Source: CAD feature listing. Evaluate the final solid. Frame: model axes, mm. Give positions to 0.01 mm unless a question says otherwise; leave off trailing zeros. Order: outer loops, then holes, each group sorted by start corner. A loop starts at its lowest first (then second) coordinate and runs counter-clockwise, first axis right, second up. Notation, with made-up numbers: (66, 66.25) -> (103, 66.25) arc R18 ccw to (103, 83.25) -> close; hole circle Ø11 at (29.5, 88.25). An arc over 180 degrees is marked (long way). Answer in a Markdown table with one row per item.
Solid Edge part; units mm, degrees
sketch "Sketch1" plane through (0, 0, 0) normal (0, 0, 1) x (1, 0, 0)
  line L0 (-52, -100) -> (52, -100)
  line L1 (52, -100) -> (52, 100)
  line L2 (52, 100) -> (-52, 100)
  line L3 (-52, 100) -> (-52, -100)
  line L4 (-25, -66) -> (25, -66)
  arc A0 (25, -66) -> (27, -64) centre (25, -64) ccw
  line L5 (27, -64) -> (27, 64)
  arc A1 (27, 64) -> (25, 66) centre (25, 64) ccw
  line L6 (25, 66) -> (-25, 66)
  arc A2 (-25, 66) -> (-27, 64) centre (-25, 64) ccw
  line L7 (-27, 64) -> (-27, -64)
  arc A3 (-25, -66) -> (-27, -64) centre (-25, -64) cw
extrude "Extrusionsausprägung_1" add sketch "Sketch1" along normal blind 2.5
hole "Bohrung_1" at (-44.9, 90, 2.5) direction (0, 0, -1) diameter 7.1 end up to next
hole "Hole1" at (44.9, 90, 2.5) direction (0, 0, -1) diameter 7.1 end up to next
hole "Hole2" at (44.9, -90, 2.5) direction (0, 0, -1) diameter 7.1 end up to next
hole "Hole3" at (-44.9, -90, 2.5) direction (0, 0, -1) diameter 7.1 end up to next
hole "Bohrung_5" at (44.9, 0, 2.5) direction (0, 0, -1) diameter 3.3 end up to next countersink diameter 6.3 countersink angle 120
hole "Hole4" at (-44.9, 0, 2.5) direction (0, 0, -1) diameter 3.3 end up to next countersink diameter 6.3 countersink angle 120
properties material "Aluminium, 2024-T4"
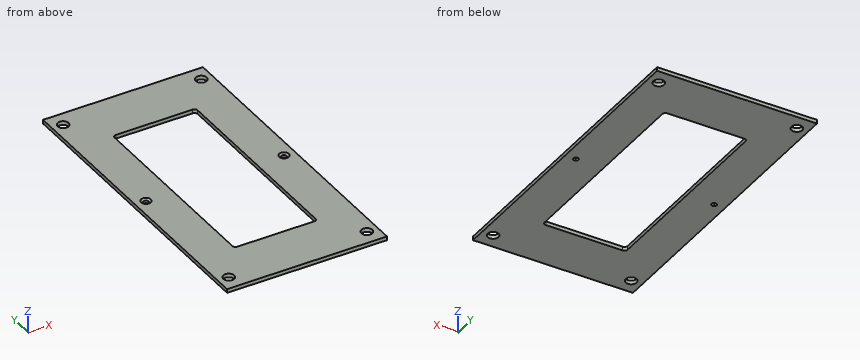
(1) Ray query, probe 1 along Y at (x, z) = (44.9, 1.3); probe 2 along X at (y, z) = (-90, 1.2); probe 3 along X at (y, z) = (0, 0.75). Return the intervals inside material, ascending.
A:
| item | result |
|---|---|
| probe 1 | y = -100 to -93.55, -86.45 to -1.65, 1.65 to 86.45, 93.55 to 100 |
| probe 2 | x = -52 to -48.45, -41.35 to 41.35, 48.45 to 52 |
| probe 3 | x = -52 to -46.55, -43.25 to -27, 27 to 43.25, 46.55 to 52 |
(2) Section query B-B (x = 5). Return the cut outline in (y, z), plus the area to 3 significant figures.
A:
| item | result |
|---|---|
| outline | (-100, 0) -> (-66, 0) -> (-66, 2.5) -> (-100, 2.5) -> close; (66, 0) -> (100, 0) -> (100, 2.5) -> (66, 2.5) -> close |
| area | 170 mm^2 |
(3) Section query D-D (y = 38). Return the cut outline in (x, z).
A:
| item | result |
|---|---|
| outline | (-52, 0) -> (-27, 0) -> (-27, 2.5) -> (-52, 2.5) -> close; (27, 0) -> (52, 0) -> (52, 2.5) -> (27, 2.5) -> close |
(4) First-contact query: pin 1 Ø4 at (x, y) = (-44.9, 0) entering from +Z. Flat tip, straight axial feed; report the tip coordinate or a pass-through.
A:
| item | result |
|---|---|
| pin 1 | stops at z = 1.84 |
(5) Section query C-C (z = 0.4). Return the cut outline in (x, y).
A:
| item | result |
|---|---|
| outline | (-52, -100) -> (52, -100) -> (52, 100) -> (-52, 100) -> close; hole circle Ø7.1 at (-44.9, -90); hole circle Ø7.1 at (-44.9, 90); hole circle Ø3.3 at (-44.9, 0); hole (-27, -64) arc R2 ccw to (-25, -66) -> (25, -66) arc R2 ccw to (27, -64) -> (27, 64) arc R2 ccw to (25, 66) -> (-25, 66) arc R2 ccw to (-27, 64) -> close; hole circle Ø7.1 at (44.9, -90); hole circle Ø7.1 at (44.9, 90); hole circle Ø3.3 at (44.9, 0) |
(6) Section query A-A (y = -90). Return the cut outline in (x, z), plus the area to 4 significant figures.
A:
| item | result |
|---|---|
| outline | (-52, 0) -> (-48.45, 0) -> (-48.45, 2.5) -> (-52, 2.5) -> close; (-41.35, 0) -> (41.35, 0) -> (41.35, 2.5) -> (-41.35, 2.5) -> close; (48.45, 0) -> (52, 0) -> (52, 2.5) -> (48.45, 2.5) -> close |
| area | 224.5 mm^2 |
